Could you check a few things on this drawing? It's one solid part, dimensions in mm from its lowest x, y, z. Give positions to 0.01 mm unless a question says otherwise; leave off trailing zeros. Order: outer loops, then holes, each group sorted by start corner. A loop starts at its lowest first (then second) coordinate and runs counter-clockwise, first axis right, second up.
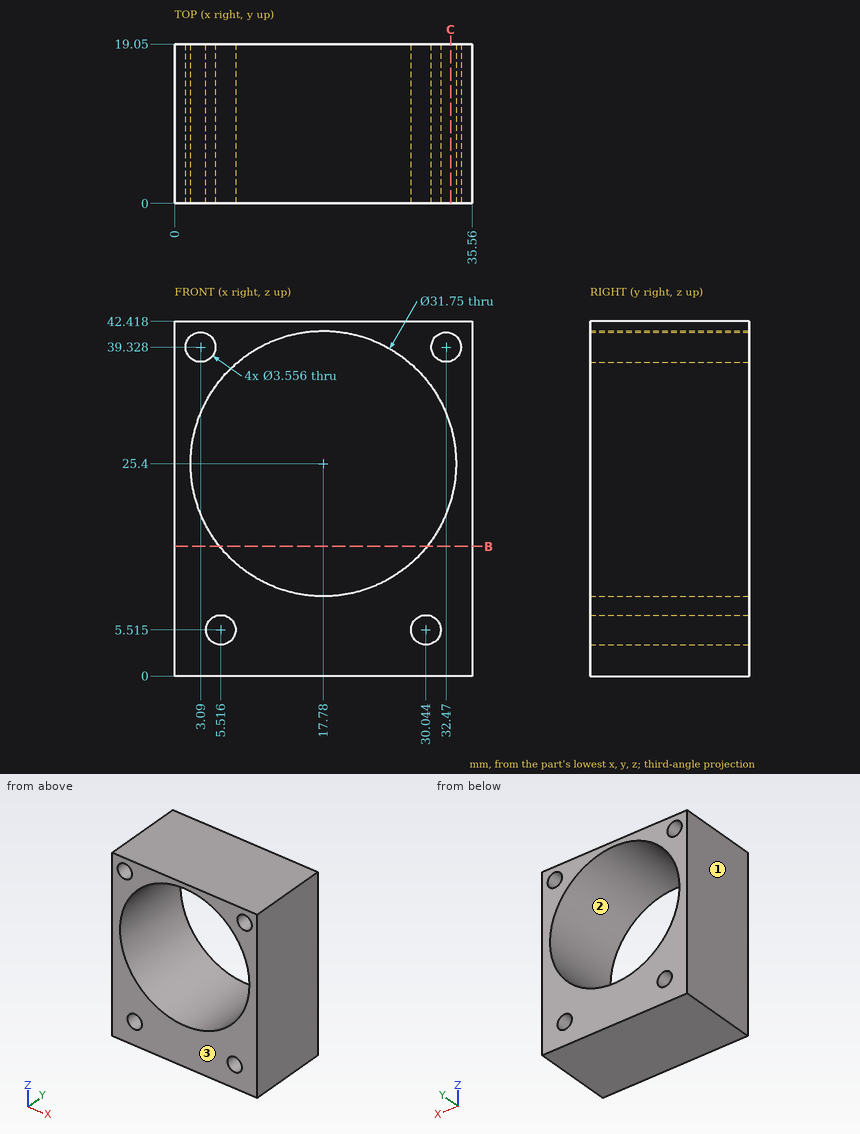
1) Suppose I cut it at B-B (z = 15.5). Please give me the cut outline in (x, y).
2) We'd pull the mould along X, two halves only. Please class the marked faces 1, 2 and 3: +X half, -X half, draft (parallel to the pull), parting line (faces both ways), or undercut.
3) Suppose I cut it at C-C (x = 33). Give the number of separate pieces and of enclosed holes in the cut face.
4) If I drill on line 1 (Z direction, x = 6, y = 10.75) (1 decimal); line 2 (Z direction, x = 31, y = 16) (1 decimal); line 3 (Z direction, x = 18, y = 16.25), over which ranges is the centre line in solid material (lowest first)?
Results:
1. outline: (0, 0) - (5.37, 0) - (5.37, 19.05) - (0, 19.05) - close; (30.19, 0) - (35.56, 0) - (35.56, 19.05) - (30.19, 19.05) - close
2. face 1: -X half
2. face 2: undercut
2. face 3: draft
3. separate pieces: 3
3. enclosed holes: 0
4. line 1: z = 0 to 3.8, 7.2 to 14.8, 36 to 42.4
4. line 2: z = 0 to 4, 7 to 16.6, 34.2 to 38.3, 40.3 to 42.4
4. line 3: z = 0 to 9.53, 41.27 to 42.42
